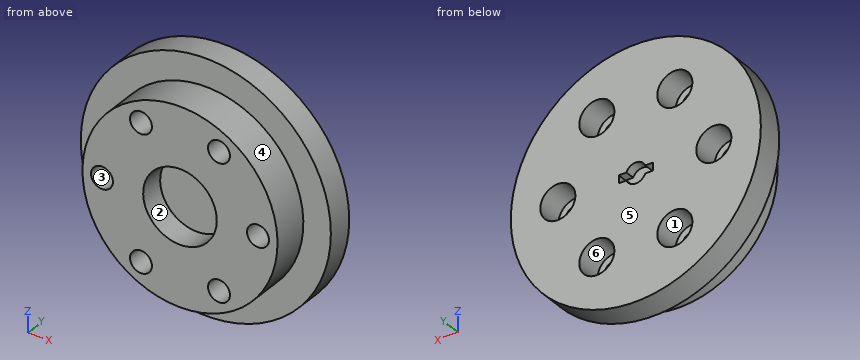
```python
from build123d import *

# Parameters (mm, degrees)
SKETCH1_R           = 20.0025
SKETCH1_R_2         = 7.55
SKETCH1_R_3         = 2.25
BOSS_EXTRUDE1_DEPTH = 7.6
SKETCH9_R           = 7.55
SKETCH9_R_2         = 6.952615
BOSS_EXTRUDE5_DEPTH = 2.6104
SKETCH2_R           = 25.64638
SKETCH2_R_2         = 3.6
BOSS_EXTRUDE2_DEPTH = 5.4
CUT_EXTRUDE1_START  = 8
SKETCH4_R           = 6.952615
CUT_EXTRUDE1_DEPTH  = 8
BOSS_EXTRUDE6_START = -8.0104
SKETCH10_R          = 6.952615
BOSS_EXTRUDE6_DEPTH = 8.0104
CUT_EXTRUDE2_DEPTH  = 2


with BuildPart() as part:
    # Sketch1 → Boss-Extrude1 (new body)
    with BuildSketch(Plane(origin=(0, 60.4104, 0), x_dir=(1, 0, 0), z_dir=(0, 1, 0))):
        with Locations(Location((0, 0, 0), (0, 0, 90))):
            Circle(SKETCH1_R)
        with Locations(Location((0, 0, 0), (0, 0, 90))):
            Circle(SKETCH1_R_2, mode=Mode.SUBTRACT)
        with Locations(Location((-8, 13.856406461, 0), (0, 0, 90))):
            Circle(SKETCH1_R_3, mode=Mode.SUBTRACT)
        with Locations(Location((8, 13.856406461, 0), (0, 0, 90))):
            Circle(SKETCH1_R_3, mode=Mode.SUBTRACT)
        with Locations(Location((16, 0, 0), (0, 0, 90))):
            Circle(SKETCH1_R_3, mode=Mode.SUBTRACT)
        with Locations(Location((8, -13.856406461, 0), (0, 0, 90))):
            Circle(SKETCH1_R_3, mode=Mode.SUBTRACT)
        with Locations(Location((-8, -13.856406461, 0), (0, 0, 90))):
            Circle(SKETCH1_R_3, mode=Mode.SUBTRACT)
        with Locations(Location((-16, 0, 0), (0, 0, 90))):
            Circle(SKETCH1_R_3, mode=Mode.SUBTRACT)
    extrude(amount=BOSS_EXTRUDE1_DEPTH)

    # Sketch9 → Boss-Extrude5 (add)
    with BuildSketch(Plane(origin=(0, 65.4, 0), x_dir=(1, 0, 0), z_dir=(0, 1, 0))):
        with Locations(Location((0, 0, 0), (0, 0, 90))):
            Circle(SKETCH9_R)
        with Locations(Location((0, 0, 0), (0, 0, 270))):
            Circle(SKETCH9_R_2, mode=Mode.SUBTRACT)
    extrude(amount=BOSS_EXTRUDE5_DEPTH)

    # Sketch2 → Boss-Extrude2 (add)
    with BuildSketch(Plane(origin=(0, 68.0104, 0), x_dir=(-1, 0, 0), z_dir=(0, -1, 0))):
        with Locations(Location((0, 0, 0), (0, 0, 180))):
            Circle(SKETCH2_R)
        with Locations(Location((-16, 0, 0), (0, 0, 180))):
            Circle(SKETCH2_R_2, mode=Mode.SUBTRACT)
        with Locations(Location((-8, 13.856406461, 0), (0, 0, 180))):
            Circle(SKETCH2_R_2, mode=Mode.SUBTRACT)
        with Locations(Location((8, 13.856406461, 0), (0, 0, 180))):
            Circle(SKETCH2_R_2, mode=Mode.SUBTRACT)
        with Locations(Location((16, 0, 0), (0, 0, 180))):
            Circle(SKETCH2_R_2, mode=Mode.SUBTRACT)
        with Locations(Location((8, -13.856406461, 0), (0, 0, 180))):
            Circle(SKETCH2_R_2, mode=Mode.SUBTRACT)
        with Locations(Location((-8, -13.856406461, 0), (0, 0, 180))):
            Circle(SKETCH2_R_2, mode=Mode.SUBTRACT)
    extrude(amount=-BOSS_EXTRUDE2_DEPTH)

    # Sketch4 → Cut-Extrude1 (cut)
    with BuildSketch(Plane.XZ.offset(-73.4104).offset(CUT_EXTRUDE1_START)):
        Circle(SKETCH4_R)
    extrude(amount=-CUT_EXTRUDE1_DEPTH, mode=Mode.SUBTRACT)

    # Sketch10 → Boss-Extrude6 (add)
    with BuildSketch(Plane(origin=(0, 73.4104, 0), x_dir=(1, 0, 0), z_dir=(0, 1, 0)).offset(BOSS_EXTRUDE6_START)):
        Circle(SKETCH10_R)
    extrude(amount=BOSS_EXTRUDE6_DEPTH)

    # Sketch11 → Cut-Extrude2 (cut)
    with BuildSketch(Plane(origin=(0, 73.4104, 0), x_dir=(1, 0, 0), z_dir=(0, 1, 0))):
        with BuildLine():
            Line((1.941648784, 0.8), (3.5, 0.8))
            Line((3.5, 0.8), (3.5, -0.8))
            Line((3.5, -0.8), (1.941648784, -0.8))
            ThreePointArc((1.941648784, -0.8), (0, -2.1), (-1.941648784, -0.8))
            Line((-1.941648784, -0.8), (-3.5, -0.8))
            Line((-3.5, -0.8), (-3.5, 0.8))
            Line((-3.5, 0.8), (-1.941648784, 0.8))
            ThreePointArc((-1.941648784, 0.8), (0, 2.1), (1.941648784, 0.8))
        make_face()
    extrude(amount=-CUT_EXTRUDE2_DEPTH, mode=Mode.SUBTRACT)


solid = part.part
```
Here's how the part is built. I have some questions about the finished solid (model axes, mm). Face numbers are marked on the shaded views. A direction names the side the tool comes from. Round coordinates to 2 decimals unless told otherwise and drop trailing zeros. Order: outer loops, then holes, each group sorted by start corner. A loop starts at its lowest first (then second) coordinate and runs counter-clockwise, first axis right, second up. Notation, with made-up numbers: (42, 84.5) -> (90, 84.5) arc R19 cw to (90, 102.5) -> close; hole circle Ø1 at (-16.75, 46). An arc over 180 degrees is marked (long way). Use a Markdown table: item, result. Add a question column.
(1) Suppose I cut it at C-C, the plane x = 0. Please give me the cut outline in (y, z).
(2) If we mould it in two halves opening along Z, with no side actions, what happens to the marked faces 4, 5 and 6? For each: released by +Z, released by -Z, zero draft, split by the parting line, or undercut.
(3) I need wall thicknesses on line 1 along X through (y, z) = (62.5, 15.5); line 2 along Z through (x, y) = (8, 66.5); line 3 along Z through (x, y) = (-8, 71.9). Which ranges of each line are inside material? Lowest first, please.
(4) For pin 1 Ø1.5 at (x, y) = (-10, 66) entering from +Z; pin 2 Ø4 at (x, z) = (16, 0) entering from +Y; pin 3 Ø0.8 at (x, y) = (-2.5, 72.5) entering from +Z; pin 4 Ø2 at (x, z) = (9.5, 15) entering from +Y, each with a flat end and sliding along its axis, tell me the tip position at first contact or that it passes through.
(5) Suppose I cut it at D-D, the plane x = 16. Please give me the cut outline in (y, z), and give its area (3 significant figures).
(6) For the marked faces 1, 2 and 3, which set-ups out of +Z, -Z, +X, -X, +Y, -Y let a thin tool reach every point of the face, with its end or its side?
(7) Suppose I cut it at A-A, the plane z = 0. Count the separate pieces of the cut face and the enclosed holes in it, and give its area (3 significant figures).
Verdict:
| question | item | result |
|---|---|---|
| 1 | outline | (60.41, -20) -> (68.01, -20) -> (68.01, -25.65) -> (73.41, -25.65) -> (73.41, -2.1) -> (71.41, -2.1) -> (71.41, 2.1) -> (73.41, 2.1) -> (73.41, 25.65) -> (68.01, 25.65) -> (68.01, 20) -> (60.41, 20) -> (60.41, 7.55) -> (65.4, 7.55) -> (65.4, -7.55) -> (60.41, -7.55) -> close |
| 2 | face 4 | split by the parting line |
| 2 | face 5 | zero draft |
| 2 | face 6 | undercut |
| 3 | line 1 | -12.64 to -9.54, -6.46 to 6.46, 9.54 to 12.64 |
| 3 | line 2 | -18.33 to -16.11, -11.61 to 11.61, 16.11 to 18.33 |
| 3 | line 3 | -24.37 to -17.46, -10.26 to 10.26, 17.46 to 24.37 |
| 4 | pin 1 | z = 17.74 |
| 4 | pin 2 | through |
| 4 | pin 3 | z = 25.56 |
| 4 | pin 4 | y = 68.01 |
| 5 | outline | (60.41, -12) -> (68.01, -12) -> (68.01, -20.04) -> (73.41, -20.04) -> (73.41, -3.6) -> (68.01, -3.6) -> (68.01, -2.25) -> (60.41, -2.25) -> close; (60.41, 2.25) -> (68.01, 2.25) -> (68.01, 3.6) -> (73.41, 3.6) -> (73.41, 20.04) -> (68.01, 20.04) -> (68.01, 12) -> (60.41, 12) -> close |
| 5 | area | 326 mm2 |
| 6 | face 1 | +Y |
| 6 | face 2 | -Y |
| 6 | face 3 | +Y, -Y |
| 7 | separate pieces | 3 |
| 7 | enclosed holes | 0 |
| 7 | area | 346 mm2 |
